Can you work these out from the drawing? Everything is in mm from the part's minimum corner. Give positions to 0.01 mm unless a question says otherwise; leave off trailing zeros. Loops run counter-clockwise (first coordinate to the right, second up) from the corner with the lowest first, then second, coordinate; pieces in that order, holes last. Notation, with made-up numbers: (71, 15.5) -> (107, 15.5) arc R20 cw to (107, 33.5) -> close; hole circle Ø11 at (-30.75, -23.75). An arc over 180 degrees is marked (long way). Write item = value, one per line. Start each with the question number.
1) I'm going to push flat-ended pins straight in: pin 1 Ø4.5 at (y, z) = (15, 15) entering from +X; pin 2 Ø8 at (x, z) = (13, 8.5) entering from +Y. Where does each tip first touch, or does it pass through?
2) I want a section at C-C (z = 15). List the corners of the cut face in (x, y) for me (3 decimals), and give its area (3 significant figures).
3) I need wall thicknesses on probe 1 along Z at (x, y) = (5.75, 15) (3 decimals); probe 2 along Y at (x, z) = (17.5, 14.5) (3 decimals); probe 3 along X at (y, z) = (13.5, 26). Which ranges of each line are inside material? Lowest first, please. Write a range as from..to.
4) I want a section at D-D (y = 15). List the corners of the cut face in (x, z) for me (1 decimal).
5) I want a section at A-A (x = 17.5). List the corners of the cut face in (y, z) for me (3 decimals), and give its area (3 significant figures).
6) I want a section at B-B (y = 10.5). List the corners of the cut face in (x, z) for me.
7) If we mould it in two halves opening along Y, with no side actions, what happens to the marked faces 1, 2 and 3? For each: +Y half, -Y half, draft (parallel to the pull), parting line (faces both ways), or undercut.
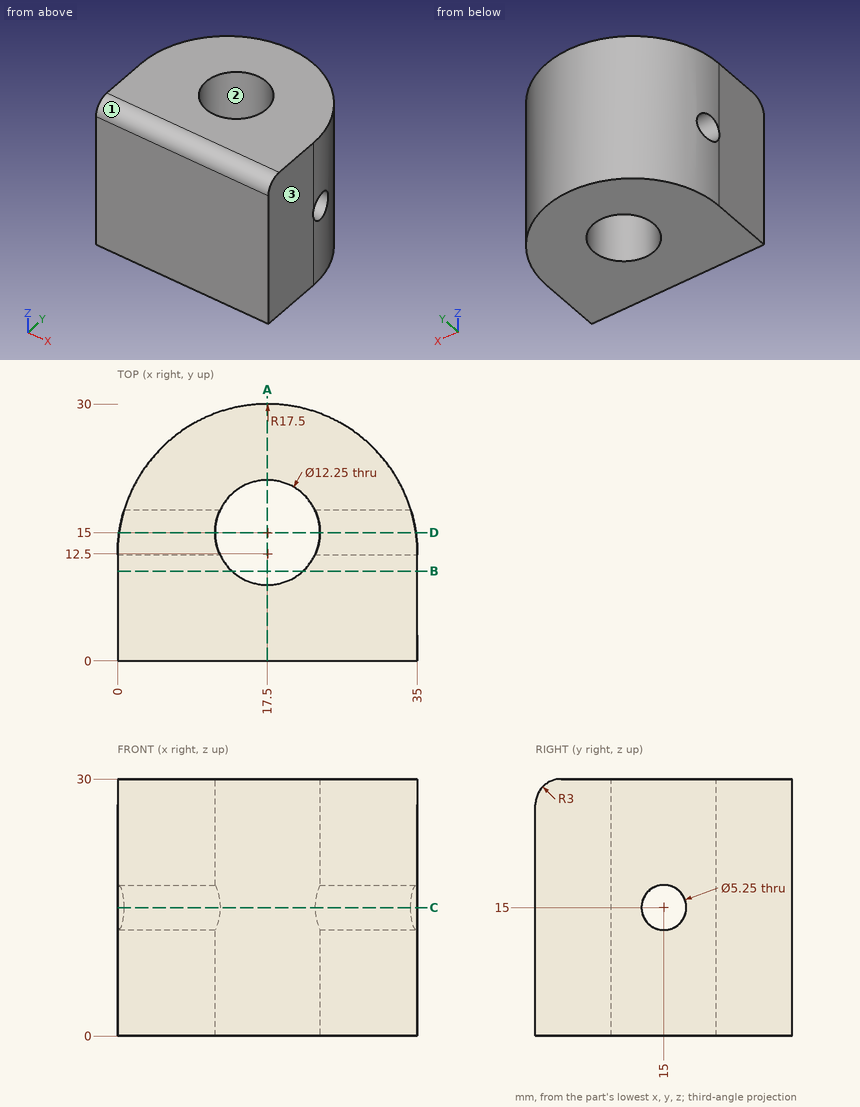
Answer list:
q1.pin_1 = through
q1.pin_2 = 29.99
q2.outline = (0, 0) -> (35, 0) -> (35, 12.375) -> (23.034, 12.375) arc R6.125 cw to (11.966, 12.375) -> (0, 12.375) -> close; (0.767, 17.625) -> (11.966, 17.625) arc R6.125 cw to (23.034, 17.625) -> (34.233, 17.625) arc R17.5 ccw to start
q2.area = 682 mm^2
q3.probe_1 = 0..12.375, 17.625..30
q3.probe_2 = 0..8.875, 21.125..30
q3.probe_3 = 0.03..11.56, 23.44..34.97
q4.outline = (0.2, 0) -> (11.4, 0) -> (11.4, 12.4) -> (0.2, 12.4) -> close; (0.2, 17.6) -> (11.4, 17.6) -> (11.4, 30) -> (0.2, 30) -> close; (23.6, 0) -> (34.8, 0) -> (34.8, 12.4) -> (23.6, 12.4) -> close; (23.6, 17.6) -> (34.8, 17.6) -> (34.8, 30) -> (23.6, 30) -> close
q5.outline = (0, 0) -> (8.875, 0) -> (8.875, 30) -> (3, 30) arc R3 ccw to (0, 27) -> close; (21.125, 0) -> (30, 0) -> (30, 30) -> (21.125, 30) -> close
q5.area = 531 mm^2
q6.outline = (0, 0) -> (13.34, 0) -> (13.34, 30) -> (0, 30) -> close; (21.66, 0) -> (35, 0) -> (35, 30) -> (21.66, 30) -> close
q7.face_1 = -Y half
q7.face_2 = undercut
q7.face_3 = draft
